Design review of the part built by this model. Coordinates are the model's own, in mm. A direction names the side the tool comes from. Round coordinates to 2 decimals unless told otherwise and drop trailing zeros. Order: outer loops, then holes, each group sorted by start corner. A loop starts at its lowest first (then second) coordinate and runs counter-clockwise, first axis right, second up. Notation, with made-up numbers: M 58.5,69.5 L 78.5,69.5 A24 ccw 78.5,84.5 Z; hole C 47.5,-4.75 d9. An arc over 180 degrees is marked long. Use a Markdown table: item, result. Add a question column.
(1) Machinability: for faces 4 (the face through (-45.353, 10.797, 2.785)), 5 (the face through (6, -19, 3.75)), 6 (the face through (-34.965, 27.216, 1.268)), which of the approach directions +Z, -Z, +X, -X, +Y, -Y give a long, thin tool a straight path to every point of the face, cutting with its end or side? Answer none if there is none.
(2) To check wall thickness, follow probe 1 along Y at (x, z) = (-11.5, 4.2); probe 2 along Y at (x, z) = (-33, 4.9); probe 3 along Y at (x, z) = (3, 1.8). State the ranges of each line that lie inside material, in increasing order. Write a range as from..to.
(3) Take a section at C-C (y = 13). Write out the cut boundary in (x, z).
(4) For pin 1 (2 mm diameter, centred on y = -15.5, z = 2, fed in from -X); pin 2 (1.8 mm diameter, centred on x = -11, y = -16.5, fed in from +Z); pin 3 (1 mm diameter, centred on y = 15, z = 3, fed in from +X), all flat-tipped, find the tip position at first contact; note any pin that passes through.
(5) The part is to be moulded in two halves that separate along X. For faces 1 (the face through (-19.15, 13.24, 2.86)), 2 (the face through (-41.801, 28.836, 2.785)), 3 (the face through (-3.67, 24.52, 2.79)), say which applies: released by +X, released by -X, zero draft, split by the parting line, or undercut.
(6) Take a section at B-B (z = 1.3). Count the separate pieces of the cut face and the enclosed holes in it, then the cut area to 3 significant figures.
(7) Take a section at A-A (y = 25). Write out the cut boundary in (x, z).
Autodesk Inventor part; units mm, degrees
ref_plane "YZ Plane" through (0, 0, 0) normal (1, 0, 0) x (0, 1, 0)
ref_plane "XZ Plane" through (0, 0, 0) normal (0, 1, 0) x (-1, 0, 0)
ref_plane "XY Plane" through (0, 0, 0) normal (0, 0, 1) x (1, 0, 0)
ref_plane "Work Plane2" through (0, 0, 0) normal (0, 0, 1) x (1, 0, 0)
sketch "Sketch1" plane through (0, 0, 0) normal (0, 0, 1) x (1, 0, 0)
  line L0 (-10, 22.5) -> (10, 22.5)
  line L1 (10, 22.5) -> (10, -22.5)
  line L2 (10, -22.5) -> (-10, -22.5)
  line L3 (-10, -22.5) -> (-10, 22.5)
  circle A0 centre (0, 17.5) radius 1.25
  circle A1 centre (5, -17.5) radius 1.25
  point P0 (0, 0)
  dimension "d38" = 20
  dimension "d39" = 45
  dimension "d40" = 2.5
  dimension "d41" = 2.5
  dimension "d42" = 10
  dimension "d43" = 5
  dimension "d44" = 5
  dimension "d45" = 5
extrude "Extrusion1" add sketch "Sketch1" along normal blind 3.65 contours L0 L1 L2 L3 | A0 | A1
sketch "Sketch2" plane through (-10, 118.2358, 3.65) normal (-1, 0, 0) x (0, 0, 1)
  line L0 (-3.65, -95.7358) -> (-3.65, -140.7358)
  line L1 (-3.65, -140.7358) -> (0, -140.7358)
  line L2 (0, -95.7358) -> (0, -140.7358)
  line L3 (-3.65, -95.7358) -> (0, -95.7358)
  point P0 (-3.65, -118.2358)
extrude "Extrusion2" add sketch "Sketch2" along normal blind 30
sketch "Sketch3" plane through (0, 0, 3.65) normal (0, 0, 1) x (1, 0, 0)
  line L0 (10, -22.5) -> (10, 22.5)
  line L1 (10, 22.5) -> (-40, 22.5)
  line L2 (-40, -22.5) -> (-40, 22.5)
  line L3 (10, -22.5) -> (-40, -22.5)
  circle A0 centre (0, 17.5) radius 3 construction
  circle A1 centre (5, -17.5) radius 3 construction
  point P0 (0, 0)
  dimension "d48" = 6
  dimension "d49" = 6
extrude "Extrusion3" add sketch "Sketch3" along normal blind 2
ref_plane "Work Plane3" through (0, 0, 0) normal (0, 0, -1) x (-1, 0, 0)
sketch "Sketch10" plane through (0, 0, 5.65) normal (0, 0, 1) x (1, 0, 0)
  circle A0 centre (-10, -17.5) radius 2.5953
  line L0 (-40, -22.5) -> (10, -22.5)
  line L1 (10, -22.5) -> (10, 22.5)
  circle A1 centre (5, -17.5) radius 2.5953
  circle A2 centre (2, 17.5) radius 2.5953
  line L2 (10, 22.5) -> (-40, 22.5)
  point P0 (0, 0)
  dimension "d75" = 5
  dimension "d76" = 20
  dimension "d77" = 8
  dimension "d78" = 5
  dimension "d79" = 5
  dimension "d80" = 5
hole "Hole4" at (-10, -17.5, 5.65) at (5, -17.5, 5.65) at (2, 17.5, 5.65) direction (0, 0, -1) diameter 3.1 end through all counterbore diameter 6 counterbore depth 1.9
sketch "Sketch11" plane through (0, 0, 5.65) normal (0, 0, 1) x (1, 0, 0)
  circle A0 centre (5, -17.5) radius 3
  circle A1 centre (-10, -17.5) radius 3
  circle A2 centre (2, 17.5) radius 3
  line L0 (-40, -22.5) -> (10, -22.5)
  line L1 (10, -22.5) -> (10, 22.5)
  line L2 (10, 22.5) -> (-40, 22.5)
  line L3 (-40, 22.5) -> (-40, -22.5)
  line L4 (-40, -22.5) -> (10, -22.5)
  line L5 (-10.1436, -22.5) -> (-40, -14.5)
  line L6 (10, 22.5) -> (-40, 22.5)
  line L7 (7, 22.5) -> (10, -11.7902)
  point P0 (0, 0)
  dimension "d81" = 15
  dimension "d82" = 8
  dimension "d83" = 5
  dimension "d84" = 3
extrude "Extrusion7" cut sketch "Sketch11" against normal through all contours L3 L5 L0 | L7 L2 L1
fillet "Fillet1" radius 5 3 edges at (10, -22.5, 2.825) (7, 22.5, 2.825) (-40, -14.5, 2.825)
sketch "Sketch12" plane through (0, 0, 5.65) normal (0, 0, 1) x (1, 0, 0)
  arc A0 (-24.0463, 1.5877) -> (-17.4606, 8.5418) centre (-23.3781, 7.5504) ccw
  arc A1 (-17.4606, 8.5418) -> (-23.6797, 15.6342) centre (-24.4593, 8.6778) ccw
  arc A2 (-30.4648, 16.3946) -> (-32.024, 2.4817) centre (-32.4095, 9.5688) ccw
  line L0 (-32.024, 2.4817) -> (-24.0463, 1.5877)
  line L1 (-23.6797, 15.6342) -> (-30.4648, 16.3946)
  point P0 (0, 0)
extrude "Extrusion8" cut sketch "Sketch12" against normal through all
sketch "Sketch13" plane through (0, 0, 0) normal (0, 0, -1) x (-1, 0, 0)
  arc A0 (32.024, 2.4817) -> (30.4648, 16.3946) centre (32.4095, 9.5688) ccw
  line L0 (32.024, 2.4817) -> (24.0463, 1.5877)
  arc A1 (17.4606, 8.5418) -> (24.0463, 1.5877) centre (23.3781, 7.5504) ccw
  arc A2 (23.6797, 15.6342) -> (17.4606, 8.5418) centre (24.4593, 8.6778) ccw
  line L1 (23.6797, 15.6342) -> (30.4648, 16.3946)
  arc A3 (36.2941, -15.493) -> (40, -10.6634) centre (35, -10.6634) ccw
  line L2 (40, 22.5) -> (40, -10.6634)
  line L3 (-2.4183, 22.5) -> (40, 22.5)
  arc A4 (-2.4183, 22.5) -> (-7.3993, 17.9358) centre (-2.4183, 17.5) ccw
  line L4 (-7.3993, 17.9358) -> (-10, -11.7902)
  line L5 (-10, -17.5) -> (-10, -11.7902)
  arc A5 (-10, -17.5) -> (-5, -22.5) centre (-5, -17.5) ccw
  line L6 (-5, -22.5) -> (10.1436, -22.5)
  line L7 (10.1436, -22.5) -> (36.2941, -15.493)
  circle A6 centre (-5, -17.5) radius 1.55
  circle A7 centre (10, -17.5) radius 1.55
  circle A8 centre (-2, 17.5) radius 1.55
  line L8 (2.3679, 22.8864) -> (2.6218, 20.62)
  line L9 (2.3679, 22.8864) -> (5.0151, 26.2019)
  line L10 (40.1666, 30.1412) -> (5.0151, 26.2019)
  line L11 (40.1666, 30.1412) -> (43.482, 27.494)
  line L12 (43.482, 27.494) -> (47.2776, -6.3746)
  line L13 (47.2776, -6.3746) -> (44.6304, -9.69)
  line L14 (44.6304, -9.69) -> (34.1957, -10.8594)
  point P0 (0, 0)
  point P1 (2.4112, 22.5)
  point P2 (40, -10.2089)
extrude "Extrusion9" add sketch "Sketch13" against normal up to surface (5.65 mm away) contours L2 L3 L8 L9 L10 L11 L12 L13 L14
sketch "Sketch14" plane through (0, 0, 0) normal (0, 0, -1) x (-1, 0, 0)
  circle A0 centre (37.6266, 25.8315) radius 1.7
  circle A1 centre (9.4116, 22.6695) radius 1.7
  circle A2 centre (10.7819, -8.452) radius 2.205
  circle A3 centre (41.5891, -4.9995) radius 1.7
  point P0 (0, 0)
hole "Hole5" at (-9.4116, 22.6695, 0) at (-37.6266, 25.8315, 0) at (-41.5891, -4.9995, 0) at (-10.7819, -8.452, 0) direction (0, 0, 1) diameter 3 end through all counterbore diameter 6 counterbore depth 2.5
properties part number "BOWDEN MOUNT"
Verdict:
| question | item | result |
|---|---|---|
| 1 | face 4 | +Z, -Z, -X, +Y |
| 1 | face 5 | +Z |
| 1 | face 6 | -Z |
| 2 | probe 1 | y = -22.14..-20.1, -14.9..-9.77, -7.14..26.93 |
| 2 | probe 2 | y = -16.38..2.5, 16.64..29.34 |
| 2 | probe 3 | y = -22.5..16.32, 18.68..22.47 |
| 3 | outline | M -45.11,0 L -38.62,0 L -38.62,5.65 L -45.11,5.65 Z; M -18.95,0 L 7.83,0 L 7.83,5.65 L -18.95,5.65 Z |
| 4 | pin 1 | stops at x = -38.21 |
| 4 | pin 2 | stops at z = 3.75 |
| 4 | pin 3 | stops at x = 7.7 |
| 5 | face 1 | undercut |
| 5 | face 2 | released by -X |
| 5 | face 3 | released by +X |
| 6 | separate pieces | 1 |
| 6 | enclosed holes | 8 |
| 6 | area | 2,070 mm^2 |
| 7 | outline | M -43.76,0 L -40.51,0 L -40.51,2.5 L -38.88,2.5 L -38.88,5.65 L -43.76,5.65 Z; M -36.38,2.5 L -34.74,2.5 L -34.74,0 L -11.3,0 L -11.3,2.5 L -7.52,2.5 L -7.52,0 L -4.06,0 L -4.06,5.65 L -36.38,5.65 Z |
